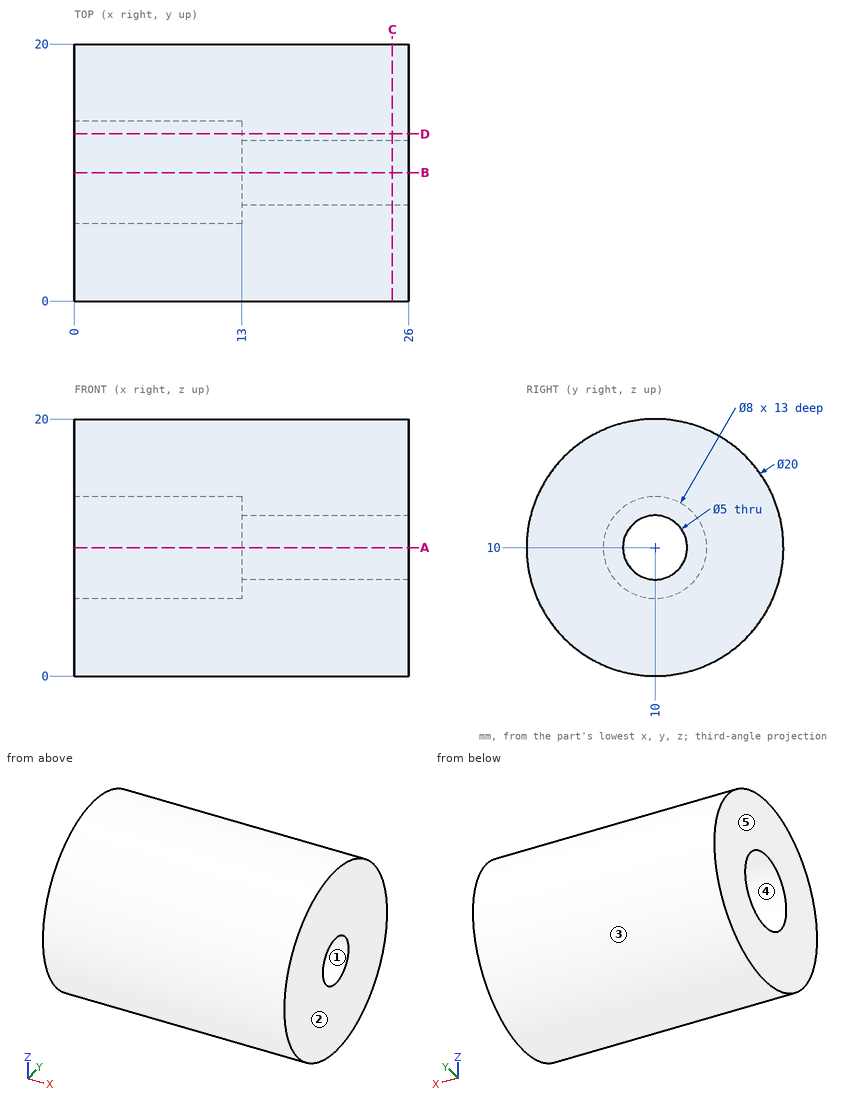
Check sheet for the drawn part. Datum: minimum x, y, z corner. Units: mm. A direction names the side the tool comes from. Give positions to 0.01 mm unless a question says otherwise; leave off trailing zeros. Order: outer loops, then holes, each group sorted by start corner. A loop starts at its lowest first (then second) coordinate and runs counter-clockwise, first axis right, second up. Notation, with made-up numbers: (84, -10) -> (98, -10) arc R15 cw to (98, 5) -> close; hole circle Ø11 at (44.5, 87.5). An arc over 180 degrees is marked (long way). Return JSON: item names as keys, results as strings.
1. Cross-section at D-D, the plane y = 13. Record the cut outline in (x, z).
From the geometry:
{"outline": "(0, 0.46) -> (26, 0.46) -> (26, 19.54) -> (0, 19.54) -> (0, 12.65) -> (13, 12.65) -> (13, 7.35) -> (0, 7.35) -> close"}
2. Material ranges on probe 1 along Y at (x, z) = (8.75, 10); probe 2 along Y at (x, z) = (4.5, 12.25); probe 3 along Z at (x, y) = (11.25, 8.75), recorded low to high. Write a range as [from, to].
From the geometry:
{"probe 1": "[0, 6], [14, 20]", "probe 2": "[0.26, 6.69], [13.31, 19.74]", "probe 3": "[0.08, 6.2], [13.8, 19.92]"}
3. Mould release check, pull along Y, two halves, no side actions. Record for the marked faces 1, 2 and 3: +Y half, -Y half, draft (parallel to the pull), parting line (faces both ways), or undercut.
From the geometry:
{"face 1": "undercut", "face 2": "draft", "face 3": "parting line"}
4. Cross-section at A-A, the plane z = 10. Record the cut outline in (x, y).
From the geometry:
{"outline": "(0, 0) -> (26, 0) -> (26, 7.5) -> (13, 7.5) -> (13, 6) -> (0, 6) -> close; (0, 14) -> (13, 14) -> (13, 12.5) -> (26, 12.5) -> (26, 20) -> (0, 20) -> close"}
5. Set-up check for the marked faces 4 and 5: record each of +Z, -Z, +X, -X, +Y, -Y from which the full face is reachable in a straight line by a thin tool's end or side.
From the geometry:
{"face 4": "-X", "face 5": "+Z, -Z, -X, +Y, -Y"}
6. Cross-section at C-C, the plane x = 24.75. Record the cut outline in (y, z), plus the area to 3 significant figures.
From the geometry:
{"outline": "circle Ø20 at (10, 10); hole circle Ø5 at (10, 10)", "area": "295 mm^2"}
7. Go/stop test with flat-tipped pins: P1, Ø1.5, axis at x = 4.5, z = 16.5, coming from the +Y side; P2, Ø2, axis at x = 17, y = 13.5, coming from the -Z side; P3, Ø1.5, axis at x = 20.5, y = 12.5, coming from the -Z side; P4, Ø3, axis at y = 10, z = 10, coming from the -X side. Record where each tip stops, or that it passes through.
From the geometry:
{"P1": "y = 18.18", "P2": "z = 0.32", "P3": "z = 0.15", "P4": "through"}
